from build123d import *

# Parameters (mm, degrees)
SKETCH1_W           = 72
SKETCH1_H           = 95
SKETCH1_R           = 2.2
SKETCH1_R_2         = 2.194279912
BOSS_EXTRUDE1_DEPTH = 10
CUT_EXTRUDE1_DEPTH  = 7
CUT_EXTRUDE2_DEPTH  = 7


with BuildPart() as part:
    # Sketch1 → Boss-Extrude1 (new body)
    with BuildSketch(Plane(origin=(0, 0, 0), x_dir=(1, 0, 0), z_dir=(0, 1, 0))):
        with Locations((117.160731424, -19.82755102)):
            Rectangle(SKETCH1_W, SKETCH1_H)
        with Locations(Location((125.160731424, 10.67244898, 0), (0, 0, 270))):
            Circle(SKETCH1_R, mode=Mode.SUBTRACT)
        with Locations(Location((109.160731424, 10.67244898, 0), (0, 0, 270))):
            Circle(SKETCH1_R, mode=Mode.SUBTRACT)
        with Locations(Location((125.160731424, -40.32755102, 0), (0, 0, 270))):
            Circle(SKETCH1_R_2, mode=Mode.SUBTRACT)
        with Locations(Location((109.160731424, -40.32755102, 0), (0, 0, 270))):
            Circle(SKETCH1_R, mode=Mode.SUBTRACT)
    extrude(amount=BOSS_EXTRUDE1_DEPTH)

    # Sketch2 → Cut-Extrude1 (cut)
    with BuildSketch(Plane.XZ):
        Polygon((109.960731424, 21.170629082), (109.960731424, 29.484472959), (117.160731424, 33.641394897), (124.360731424, 29.484472959), (124.360731424, 21.170629082), (117.160731424, 17.013707144), align=None)
    extrude(amount=-CUT_EXTRUDE1_DEPTH, mode=Mode.SUBTRACT)

    # Sketch5 → Cut-Extrude2 (cut)
    with BuildSketch(Plane.XZ.offset(-7)):
        with BuildLine():
            ThreePointArc((121.360731424, 25.32755102), (120.130579905, 28.297399501), (117.160731424, 29.52755102))
            Line((117.160731424, 29.52755102), (117.160731424, 21.12755102))
            ThreePointArc((117.160731424, 21.12755102), (120.130579905, 22.357702539), (121.360731424, 25.32755102))
        make_face()
        with BuildLine():
            Line((117.160731424, 21.12755102), (117.160731424, 29.52755102))
            ThreePointArc((117.160731424, 29.52755102), (112.960731424, 25.32755102), (117.160731424, 21.12755102))
        make_face()
    extrude(amount=-CUT_EXTRUDE2_DEPTH, mode=Mode.SUBTRACT)


solid = part.part
The model under review builds one solid part; all positions refer to its coordinate system, in mm. A direction names the side the tool comes from. Coordinates: 2 decimals unless noted, no trailing zeros. Write each loop counter-clockwise with the first axis right and the second up, starting at its lowest first coordinate (ties: lowest second). Pieces come first, ordered by that corner, then holes. Notation, with made-up numbers: (18.5, 68.25) - (73.5, 68.25) arc R21 ccw to (73.5, 99.25) - close; hole circle Ø7 at (54, -5). An arc over 180 degrees is marked (long way). Answer as a JSON object with one key per item and string values. Group by question number.
1. Mouldability with a two-part tool opening along Z and no side actions: class faces 3 (the face through (153.161, 5, 20)), 4 (the face through (117, 5, -27.672)), 5 (the face through (127.016, 4.93, -9.49)), 6 (the face through (109.961, 3, 25)) as pulls with the +Z half, pulls with the -Z half, needs draft (parallel to the pull), parting line crosses it, or undercut.
2. Machinability: for faces 1 (the face through (124.361, 3, 25)), 2 (the face through (117, 10, 19)), which of the approach directions +Z, -Z, +X, -X, +Y, -Y give a long, thin tool a straight path to every point of the face, cutting with its end or side? Answer none if there is none.
3. Add section B-B (y = 1.5). Give the boundary of the cut face in (x, z).
4. To check wall thickness, follow probe 1 along Z at (x, y) = (127, 1.5); probe 2 along Y at (x, z) = (122, 26); probe 3 along Z at (x, y) = (111.5, 1). State the ranges of each line that lie inside material, in increasing order.
5. Add section A-A (z = -10). Give the boundary of the cut face in (x, y), plus the area to 3 significant figures.
6. Clearance check with flat-ended pins moving along their axes: pin 1 Ø5 at (x, z) = (136, 47) entering from -Y; pin 2 Ø4.5 at (x, z) = (119.5, 29.5) entering from -Y. State where each tip first meets the part, or that it passes through.
7. Add section C-C (z = 18). Give the boundary of the cut face in (x, y).
Findings:
{
 "1": {"face 3": "needs draft", "face 4": "pulls with the -Z half", "face 5": "undercut", "face 6": "undercut"},
 "2": {"face 1": "-Y", "face 2": "+Z, -Z, +X, -X, +Y"},
 "3": {"outline": "(81.16, -27.67) - (153.16, -27.67) - (153.16, 67.33) - (81.16, 67.33) - close; hole circle Ø4.4 at (109.16, -10.67); hole circle Ø4.4 at (109.16, 40.33); hole (109.96, 21.17) - (117.16, 17.01) - (124.36, 21.17) - (124.36, 29.48) - (117.16, 33.64) - (109.96, 29.48) - close; hole circle Ø4.4 at (125.16, -10.67); hole circle Ø4.39 at (125.16, 40.33)"},
 "4": {"probe 1": "-27.67 to -11.88, -9.47 to 39.13, 41.52 to 67.33", "probe 2": "7 to 10", "probe 3": "-27.67 to 20.28, 30.37 to 67.33"},
 "5": {"outline": "(81.16, 0) - (107.07, 0) - (107.07, 10) - (81.16, 10) - close; (111.26, 0) - (123.07, 0) - (123.07, 10) - (111.26, 10) - close; (127.26, 0) - (153.16, 0) - (153.16, 10) - (127.26, 10) - close", "area": "636 mm²"},
 "6": {"pin 1": "y = 0", "pin 2": "y = 7"},
 "7": {"outline": "(81.16, 0) - (115.45, 0) - (115.45, 7) - (118.87, 7) - (118.87, 0) - (153.16, 0) - (153.16, 10) - (81.16, 10) - close"}
}
